Design review of the part built by this model. Coordinates are the model's own, in mm. A direction names the side the tool comes from. Give positions to 0.01 mm unless a question says otherwise; leave off trailing zeros. Write each loop counter-clockwise with the first axis right and the second up, starting at its lowest first coordinate (ties: lowest second). Pieces come first, ordered by that corner, then holes. Notation, with made-up numbers: (-12, 88.5) - (12, 88.5) arc R16 ccw to (12, 109.5) - close; hole circle Ø3 at (28, 71). An arc over 180 degrees is marked (long way). Use a Markdown table: item, result. Add a question column.
Autodesk Inventor part; units mm, degrees
ref_plane "YZ Plane" through (0, 0, 0) normal (1, 0, 0) x (0, 1, 0)
ref_plane "XZ Plane" through (0, 0, 0) normal (0, 1, 0) x (-1, 0, 0)
ref_plane "XY Plane" through (0, 0, 0) normal (0, 0, 1) x (1, 0, 0)
sketch "Sketch1" plane through (0, 0, 0) normal (1, 0, 0) x (0, 1, 0)
  line L0 (16.8586, 5.2751) -> (-11.0014, 5.2751)
  line L1 (-11.0014, 5.2751) -> (-11.0014, -13.7249)
  line L2 (-11.0014, -13.7249) -> (16.8586, -13.7249)
  line L3 (16.8586, -13.7249) -> (16.8586, 5.2751)
  line L4 (-2.1014, 5.2751) -> (-2.1014, -13.7249)
  line L5 (-4.0014, 5.2751) -> (-4.0014, -13.7249)
  point P0 (0, 0)
  point P1 (12.3586, -4.2249)
  point P2 (-7.8914, -4.2249)
  dimension "d1" = 19
  dimension "d2" = 1.9
  dimension "d3" = 18.96
  dimension "d4" = 7
  dimension "d19" = 9.5
  dimension "d39" = 20.25
  dimension "d40" = 4.5
extrude "Extrusion1" add sketch "Sketch1" along normal blind 8.5 contours L3 L2 L4 L0 | L5 L2 L1 L0
sketch "Sketch2" plane through (8.5, 0, 0) normal (1, 0, 0) x (0, 0, -1)
  line L0 (-5.2751, 16.8586) -> (-5.2751, -2.1014)
  line L1 (-5.2751, -2.1014) -> (13.7249, -2.1014)
  line L2 (13.7249, -2.1014) -> (13.7249, 16.8586)
  line L3 (13.7249, 16.8586) -> (-5.2751, 16.8586)
  line L4 (13.7249, -11.0014) -> (13.7249, -4.0014)
  line L5 (13.7249, -4.0014) -> (-5.2751, -4.0014)
  line L6 (-5.2751, -4.0014) -> (-5.2751, -11.0014)
  line L7 (-5.2751, -11.0014) -> (13.7249, -11.0014)
  line L8 (-5.2751, -2.1014) -> (-5.2751, -4.0014)
  line L9 (13.7249, -2.1014) -> (13.7249, 16.8586)
  line L10 (13.7249, -11.0014) -> (13.7249, -4.0014)
  line L11 (13.7249, -2.1014) -> (13.7249, -4.0014)
  point P0 (0, 0)
extrude "Extrusion2" add sketch "Sketch2" along normal blind 2
sketch "Sketch3" plane through (0, 0, 0) normal (-1, 0, 0) x (0, 0, 1)
  line L0 (-13.7249, -11.0014) -> (-13.7249, -4.0014)
  line L1 (5.2751, -11.0014) -> (-13.7249, -11.0014)
  line L2 (5.2751, -4.0014) -> (5.2751, -11.0014)
  line L3 (-13.7249, -4.0014) -> (5.2751, -4.0014)
  line L4 (5.2751, 16.8586) -> (5.2751, -2.1014)
  line L5 (-13.7249, 16.8586) -> (5.2751, 16.8586)
  line L6 (-13.7249, -2.1014) -> (-13.7249, 16.8586)
  line L7 (5.2751, -2.1014) -> (-13.7249, -2.1014)
  line L8 (-12.6249, -4.0014) -> (-11.8249, -4.0014)
  line L9 (-11.8249, -4.0014) -> (-11.8249, -3.0014)
  line L10 (-11.8249, -3.0014) -> (-12.6249, -3.0014)
  line L11 (-12.6249, -3.0014) -> (-12.6249, -4.0014)
  point P0 (0, 0)
  dimension "d9" = 1
  dimension "d10" = 0.8
  dimension "d11" = 1.1
extrude "Extrusion3" add sketch "Sketch3" against normal up to surface (8.5 mm away) contours L11 L10 L9 L3
fillet "Fillet1" radius 0.2 2 edges at (4.25, -3.0014, -12.6249) (4.25, -3.0014, -11.8249)
pattern_linear "Rectangular Pattern1" count 9 spacing 2 along (0, 0, 1) of "Extrusion3", "Fillet1"
hole "Hole2" at (0, 12.3586, -4.2249) at (0, -7.8914, -4.2249) direction (1, 0, 0) diameter 3 end through all
fillet "Fillet3" radius 3 2 edges at (5.25, -11.0014, -13.7249) (5.25, -11.0014, 5.2751)
fillet "Fillet3" radius 2 2 edges at (5.25, 16.8586, 5.2751) (5.25, 16.8586, -13.7249)
sketch "Sketch4" plane through (0, 16.8586, 3.2751) normal (0, 1, 0) x (1, 0, 0)
  line L0 (0, 15) -> (10.5, 15)
  line L1 (0, 15) -> (0, 0)
  line L2 (10.5, 0) -> (0, 0)
  line L3 (10.5, 15) -> (10.5, 0)
  line L4 (10.5, 17) -> (10.5, 15)
  line L5 (10.5, 15) -> (30.5, 15)
  line L6 (30.5, 15) -> (30.5, 0)
  line L7 (30.5, 0) -> (10.5, 0)
  line L8 (30.5, 11.5) -> (40.5, 11.5)
  line L9 (40.5, 11.5) -> (40.5, 3.5)
  line L10 (40.5, 3.5) -> (30.5, 3.5)
  point P0 (0, 3.2751)
  dimension "d50" = 20
  dimension "d51" = 15
  dimension "d52" = 8
  dimension "d53" = 3.5
  dimension "d54" = 10
extrude "Extrusion4" add sketch "Sketch4" along normal blind 10
chamfer "Chamfer4" distance 20 distance2 3.5 1 edges at (30.5, 21.8586, 3.2751) measured on face at (13.6667, 23.5253, 3.2751)
chamfer "Chamfer5" distance 20 distance2 3.5 1 edges at (30.5, 21.8586, -11.7249) measured on face at (13.6667, 23.5253, -11.7249)
chamfer "Chamfer6" distance 30 distance2 4 1 edges at (40.5, 26.8586, -4.2249) measured on face at (17.167, 26.8586, -2.8915)
fillet "Fillet4" radius 2 4 edges at (5.25, 16.8586, 3.2751) (5.25, 26.8586, 3.2751) (5.25, 26.8586, -11.7249) (5.25, 16.8586, -11.7249)
fillet "Fillet4" radius 3 1 edges at (10.5, 16.8586, -4.2249)
sketch "Sketch5" plane through (10.5, -8.0014, 5.2751) normal (1, 0, 0) x (0, 0, -1)
  line L0 (2, 26.3241) -> (2, 21.86)
  arc A0 (1, 24.5921) -> (2, 26.3241) centre (0, 26.3241) ccw
  arc A1 (1, 24.5921) -> (0, 22.86) centre (2, 22.86) ccw
  line L1 (0, 22.86) -> (0, 0)
  arc A2 (0, 0) -> (3, -3) centre (3, 0) ccw
  line L2 (3, -3) -> (16, -3)
  arc A3 (16, -3) -> (19, 0) centre (16, 0) ccw
  line L3 (19, 0) -> (19, 22.86)
  arc A4 (19, 22.86) -> (18, 24.5921) centre (17, 22.86) ccw
  arc A5 (17, 26.3241) -> (18, 24.5921) centre (19, 26.3241) ccw
  line L4 (17, 21.86) -> (17, 26.3241)
  line L5 (9.5, 21.86) -> (17, 21.86)
  circle A6 centre (9.5, 20.36) radius 1.5
  line L6 (2, 21.86) -> (9.5, 21.86)
  circle A7 centre (9.5, 0.11) radius 1.5
  circle A8 centre (9.5, 20.36) radius 1.5
  circle A9 centre (9.5, 20.36) radius 3
  point P0 (5.2751, 8.0014)
  dimension "d68" = 6
extrude "Extrusion5" cut sketch "Sketch5" along normal blind 10 contours A9 L5 L6 | L6 L5 A9
sketch "Sketch6" plane through (30.5, 16.8586, -0.2249) normal (0, 0, 1) x (1, 0, 0)
  point P0 (-30.5, -16.8586)
equation "\"d53\" = -0.5 * d52 + 0.5 * d51"
properties part number "3DP_PLA_X_axis_carriage_belt_mount" material "ABS Plastic"
(1) Insertion check: pin 1 (4 mm diameter, centred on y = 9.5, z = -7, fed in from +X); pin 2 (8 mm diameter, centred on x = 36, y = 20.5, fed in from +Z); pin 3 (8 mm diameter, centred on x = 17, y = 8, fed in from +Z); pin 4 (0.9 mm diameter, centred on x = 3, y = -3.5, fed in from -Z). Each pin has a flat end and moves straight along its axis. Give the tip position at first contact, or say it passes through.
(2) Mouldability with a two-part tool opening along Y and no side actions: class faces 1 (the face through (22.377, 25.275, -4.321)), 2 (the face through (5.32, -10.1, 4.42)), 3 (the face through (4, -4.001, -7)), 4 (the face through (10.5, 1, -4)) as +Y half, -Y half, draft (parallel to the pull), parting line (faces both ways), or undercut.
(3) Add section A-A (x = 6). Count the separate pieces of the cut face and the enclosed holes in it, and give its area (3 significant figures).
(4) Tool access review of faces 5 (the face through (8.5, -2.8, -2)), 6 (the face through (4, -4.001, 5)), 7 (the face through (36, 20, -0.225)), 8 (the face through (5, 22, 3.275)): name each direction out of +Z, -Z, +X, -X, +Y, -Y from which nothing blocks a thin tool from reaching the whole face with its end or side.
(5) Add section B-B (y = 4). State the section outline as (x, z) points, and give its area (4 significant figures).
(6) For line 1 along Y through (x, z) = (5.5, -0.75); line 2 along X through (y, z) = (10, 0); line 3 along Z through (x, y) = (7.5, 15), list the stretches that pass through material, from the lowest coordinate up.
(7) Add section C-C (x = 15). State the section outline as (y, z) points.
Answers follow:
| question | item | result |
|---|---|---|
| 1 | pin 1 | x = 10.5 |
| 1 | pin 2 | z = -0.22 |
| 1 | pin 3 | through |
| 1 | pin 4 | z = -12.62 |
| 2 | face 1 | +Y half |
| 2 | face 2 | -Y half |
| 2 | face 3 | undercut |
| 2 | face 4 | draft |
| 3 | separate pieces | 2 |
| 3 | enclosed holes | 2 |
| 3 | area | 629 mm^2 |
| 4 | face 5 | -X |
| 4 | face 6 | +Z, -X |
| 4 | face 7 | +Z, +X, +Y, -Y |
| 4 | face 8 | +Z, +X, -X, +Y |
| 5 | outline | (0, -13.72) - (10.5, -13.72) - (10.5, 5.28) - (0, 5.28) - close |
| 5 | area | 199.5 mm^2 |
| 6 | line 1 | -11 to -4, -2.1 to 26.86 |
| 6 | line 2 | 0 to 10.5 |
| 6 | line 3 | -13.72 to 5.27 |
| 7 | outline | (16.86, -10.94) - (26.26, -10.94) - (26.26, 2.49) - (16.86, 2.49) - close |
